Verification items for the finished model (mm, model axes). Round coordinates to 2 decimals unless told otherwise and drop trailing zeros. Write each loop counter-clockwise with the first axis right and the second up, starting at its lowest first coordinate (ties: lowest second). Pieces come first, ordered by that corner, then holes. Notation, with made-up numbers: (65.25, -14) - (81.25, -14) arc R29 cw to (81.25, 19) - close; hole circle Ø10 at (44.25, 26). An arc over 180 degrees is marked (long way). Answer as a JSON object with one key per item and string values.
```python
from build123d import *

# Parameters (mm, degrees)
SKETCH_2_R      = 3.85
EXTRUDE_1_DEPTH = 1.5


with BuildPart() as part:
    # 草圖2 → 填料-伸長1 (new body)
    with BuildSketch(Plane(origin=(0, 0, 0), x_dir=(0, 0, -1), z_dir=(1, 0, 0))):
        with BuildLine():
            Line((86.867278103, 6.136277943), (-86.867278103, 6.136277943))
            ThreePointArc((-86.867278103, 6.136277943), (-93.10532064, 7.340711326), (-98.653191396, 10.436670715))
            ThreePointArc((-98.653191396, 10.436670715), (-120.185454546, 0), (-98.653191396, -10.436670715))
            ThreePointArc((-98.653191396, -10.436670715), (-93.10532064, -7.340711326), (-86.867278103, -6.136277943))
            Line((-86.867278103, -6.136277943), (86.867278103, -6.136277943))
            ThreePointArc((86.867278103, -6.136277943), (93.10532064, -7.340711326), (98.653191396, -10.436670715))
            ThreePointArc((98.653191396, -10.436670715), (120.185454546, 0), (98.653191396, 10.436670715))
            ThreePointArc((98.653191396, 10.436670715), (93.10532064, 7.340711326), (86.867278103, 6.136277943))
        make_face()
        with Locations((-106.89, 0)):
            Circle(SKETCH_2_R, mode=Mode.SUBTRACT)
        with Locations((106.89, 0)):
            Circle(SKETCH_2_R, mode=Mode.SUBTRACT)
    extrude(amount=EXTRUDE_1_DEPTH)


solid = part.part
```
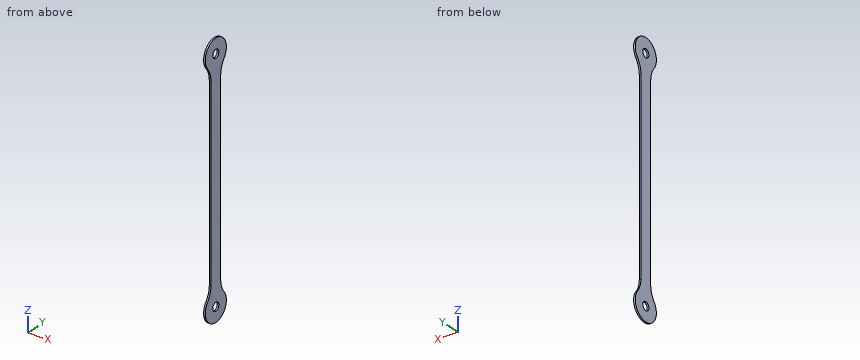
Q1. Material ranges on line 1 along Z through (x, y) = (1.4, -1.75); line 2 along Y through (x, z) = (0.4, 106.89); line 3 along Y through (x, z) = (0.15, -69.5), recorded low to high. Write a range as [from, to].
Geometry check:
{"line 1": "z = [-120.07, -110.32], [-103.46, 103.46], [110.32, 120.07]", "line 2": "y = [-13.3, -3.85], [3.85, 13.3]", "line 3": "y = [-6.14, 6.14]"}
Q2. Section check C-C, the plane x = 1.25. Record the cut outline in (y, z).
Geometry check:
{"outline": "(-10.44, -98.65) arc R13.3 ccw (long way) to (10.44, -98.65) arc R20.05 cw to (6.14, -86.87) - (6.14, 86.87) arc R20.05 cw to (10.44, 98.65) arc R13.3 ccw (long way) to (-10.44, 98.65) arc R20.05 cw to (-6.14, 86.87) - (-6.14, -86.87) arc R20.05 cw to start; hole circle Ø7.7 at (0, -106.89); hole circle Ø7.7 at (0, 106.89)"}
Q3. Section check D-D, the plane z = -21. Record the cut outline in (x, y).
Geometry check:
{"outline": "(0, -6.14) - (1.5, -6.14) - (1.5, 6.14) - (0, 6.14) - close"}
Q4. Gauge pin test, flat ends, axial feed: P1, Ø3, axis at y = -2, z = 30, coming from the -X side; P2, Ø0.8, axis at x = 0.5, z = 6, coming from the -Y side. Record the tip position at first contact, or that the pin passes through.
Geometry check:
{"P1": "stops at x = 0", "P2": "stops at y = -6.14"}
Q5. Section check A-A, the plane y = 0. Record the cut outline in (x, z), then the cut area to 3 significant figures.
Geometry check:
{"outline": "(0, -120.19) - (1.5, -120.19) - (1.5, -110.74) - (0, -110.74) - close; (0, -103.04) - (1.5, -103.04) - (1.5, 103.04) - (0, 103.04) - close; (0, 110.74) - (1.5, 110.74) - (1.5, 120.19) - (0, 120.19) - close", "area": "337 mm2"}
Q6. Section check B-B, the plane z = -106.89. Record the cut outline in (x, y).
Geometry check:
{"outline": "(0, -13.3) - (1.5, -13.3) - (1.5, -3.85) - (0, -3.85) - close; (0, 3.85) - (1.5, 3.85) - (1.5, 13.3) - (0, 13.3) - close"}
